Design review of the part shown in the three views and the two pictorial views. Dimensions are in mm from the part's minimum x, y and z. A direction names the side the tool comes from. Round coordinates to 2 decimals unless told otherwise and drop trailing zeros. Loops run counter-clockwise (first coordinate to the right, second up) from the corner with the lowest first, then second, coordinate; pieces in that order, holes last. Notation, with made-up numbers: (-33.75, 86.5) -> (17.25, 86.5) arc R12 ccw to (17.25, 97.5) -> close; hole circle Ø3 at (10, 64.5). An arc over 180 degrees is marked (long way). Write each question's results on one line, items separated by ' | '. Start each with the question number.
Item 1: For L1, parallel to Z at x = 82.5, y = 13; L2, parallel to Z at x = 48, y = 53.5; L3, parallel to X at y = 54, z = 30.5 (1 decimal), list the stretches that pass through material, from the lowest coordinate up. Write a range as from..to.
Item 2: We need section A-A (y = 43.5). Give the boundary of the cut face in (x, z).
Item 3: We need section C-C (z = 32). Give the boundary of the cut face in (x, y) (1 decimal).
Item 4: We need section D-D (y = 12.5). Give the boundary of the cut face in (x, z), and give its area (3 significant figures).
Item 5: Clearance check with flat-ended pins moving along their axes: pin 1 Ø12 at (x, z) = (83, 21.5) entering from -Y; pin 2 Ø6 at (x, z) = (49, 33) entering from -Y; pin 3 Ø5 at (x, y) = (57, 53) entering from +Z (1 decimal); pin 4 Ø1 at (y, z) = (29.5, 28) entering from +X. State where each tip first meets the part, or that it passes through.
Item 6: Tool access review of the marked faces 1 and 2: name each direction out of +Z, -Z, +X, -X, +Y, -Y from which nothing blocks a thin tool from reaching the whole face with its end or side.
Item 7: We need section B-B (x = 92). Give the boundary of the cut face in (y, z), and give its area (3 significant figures).
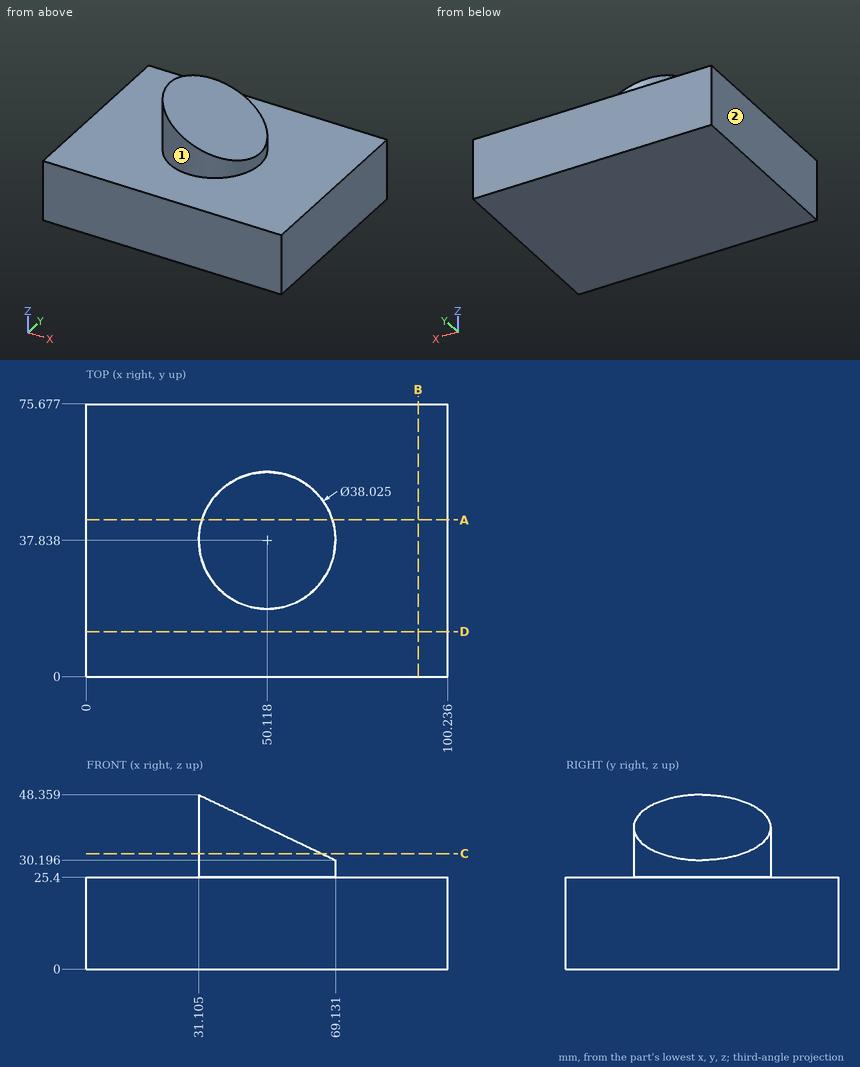
Here are the results:
1) L1: z = 0..25.4 | L2: z = 0..40.29 | L3: x = 40.1..60.1
2) outline: (0, 0) -> (100.24, 0) -> (100.24, 25.4) -> (68.27, 25.4) -> (68.27, 30.61) -> (31.97, 47.95) -> (31.97, 25.4) -> (0, 25.4) -> close
3) outline: (65.4, 26.5) -> (65.4, 49.2) arc R19 ccw (long way) to start
4) outline: (0, 0) -> (100.24, 0) -> (100.24, 25.4) -> (0, 25.4) -> close | area: 2,550 mm2
5) pin 1: stops at y = 0 | pin 2: stops at y = 18.83 | pin 3: stops at z = 37.2 | pin 4: stops at x = 67.44
6) face 1: +Z | face 2: +Z, -Z, -X, +Y, -Y
7) outline: (0, 0) -> (75.68, 0) -> (75.68, 25.4) -> (0, 25.4) -> close | area: 1,920 mm2
